The listing builds one solid part. Answer for the finished solid, in the listing's coordinates (mm). A direction names the side the tool comes from. Round coordinates to 2 decimals unless told otherwise and drop trailing zeros. Loops run counter-clockwise (first coordinate to the right, second up) from the corner with the lowest first, then second, coordinate; pieces in that order, holes last. Notation, with made-up numbers: M -9.75,49 L 48.25,49 A13 ccw 48.25,57 Z; hole C 55,71 d4. An arc over 180 degrees is marked long. Answer as a JSON object with one key per item and string values.
```python
from build123d import *

# Parameters (mm, degrees)
F1_DEPTH       = 10
F3_D           = 3.7973
F3_CSINK_D     = 7.7978
F3_CSINK_ANGLE = 82
F4_SIZE        = 5
F5_R           = 5
F6_R           = 15


with BuildPart() as f1:
    # F0 (on Front) → F1 (new body, symmetric)
    with BuildSketch(Plane.XZ):
        with BuildLine():
            Line((0, -15), (0, 15))
            ThreePointArc((0, 15), (-2.4851818051, 16.4611506644), (-5, 17.8706822588))
            Line((-5, 17.8706822588), (-5, 14.2103387279))
            Line((-5, 14.2103387279), (-5, -14.2103387279))
            Line((-5, -14.2103387279), (-5, -17.8706822588))
            ThreePointArc((-5, -17.8706822588), (-2.4851818051, -16.4611506644), (0, -15))
        make_face()
        with BuildLine():
            Line((0, 15), (0, 65))
            Line((0, 65), (-5, 65))
            Line((-5, 65), (-5, 17.8706822588))
            ThreePointArc((-5, 17.8706822588), (-2.4851818051, 16.4611506644), (0, 15))
        make_face()
        with BuildLine():
            Line((0, -65), (0, -15))
            ThreePointArc((0, -15), (-2.4851818051, -16.4611506644), (-5, -17.8706822588))
            Line((-5, -17.8706822588), (-5, -65))
            Line((-5, -65), (0, -65))
        make_face()
        with BuildLine():
            Line((-5, 14.2103387279), (-5, 17.8706822588))
            ThreePointArc((-5, 17.8706822588), (-72.3928986571, 34.9994712149), (-139.6904967398, 17.5))
            ThreePointArc((-139.6904967398, 17.5), (-147.231014529, 10.1554893712), (-150, 0))
            ThreePointArc((-150, 0), (-147.231014529, -10.1554893712), (-139.6904967398, -17.5))
            ThreePointArc((-139.6904967398, -17.5), (-72.3928986571, -34.9994712149), (-5, -17.8706822588))
            Line((-5, -17.8706822588), (-5, -14.2103387279))
            ThreePointArc((-5, -14.2103387279), (-71.5057739854, -31.7990733195), (-138.1393945883, -14.7010569646))
            ThreePointArc((-138.1393945883, -14.7010569646), (-144.4738849633, -8.5312244428), (-146.8, 0))
            ThreePointArc((-146.8, 0), (-144.4738849633, 8.5312244428), (-138.1393945883, 14.7010569646))
            ThreePointArc((-138.1393945883, 14.7010569646), (-71.5057739854, 31.7990733195), (-5, 14.2103387279))
        make_face()
    extrude(amount=F1_DEPTH, both=True)

    # F3 (through all)
    with Locations(Plane(origin=(-5, 0, 0), x_dir=(0, -1, 0), z_dir=(-1, 0, 0))):
        with Locations((0, 55), (0, -55)):
            CounterSinkHole(F3_D / 2, F3_CSINK_D / 2, counter_sink_angle=F3_CSINK_ANGLE)

    # F4
    f4_edges = [f1.edges().sort_by_distance(p)[0] for p in [
        (-2.5, -10, 65),
        (-2.5, 10, 65),
        (-2.5, -10, -65),
        (-2.5, 10, -65),
    ]]
    chamfer(f4_edges, length=F4_SIZE)

    # F5
    f5_edges = [f1.edges().sort_by_distance(p)[0] for p in [
        (-2.5, -5, -65),
        (-2.5, 5, -65),
        (-2.5, -5, 65),
        (-2.5, 5, 65),
    ]]
    fillet(f5_edges, radius=F5_R)

    # F6
    f6_edges = [f1.edges().sort_by_distance(p)[0] for p in [
        (-5, 0, 14.210339),
        (-5, 0, 17.870682),
        (-5, 0, -17.870682),
        (-5, 0, -14.210339),
    ]]
    fillet(f6_edges, radius=F6_R)


solid = f1.part
```
Item 1: The part is cut by section A-A (z = -55). Give the vertices of the cut face in (x, y), then the cut area to 3 significant figures.
Values follow:
{"outline": "M -5,-10 L 0,-10 L 0,-1.9 L -2.7,-1.9 L -5,-3.9 Z; M -5,3.9 L -2.7,1.9 L 0,1.9 L 0,10 L -5,10 Z", "area": "76.4 mm^2"}
Item 2: Flat-ended cylindrical pins translate along their axes: P1, Ø8, axis at y = 6.5, z = -12, coming from the -X side; P2, Ø8, axis at y = -2.5, z = -51, coming from the -X side; P3, Ø6, axis at y = -6, z = 5, coming from the -X side. Find the tip coordinate at first contact, or state that the pin passes through.
Values follow:
{"P1": "x = -148.33", "P2": "x = -5", "P3": "x = -149.9"}
Item 3: The part is cut by section B-B (x = -19). Give the vertices of the cut face in (y, z).
Values follow:
{"outline": "M -10,-26.02 L 10,-26.02 L 10,-21.08 L -10,-21.08 Z; M -10,21.08 L 10,21.08 L 10,26.02 L -10,26.02 Z"}
Item 4: Determine the mould class of faces 4 (the face through (-84.204, -0.14, -34.466)), 5 (the face through (-7.26, 0.14, 13.02)), 6 (the face through (-11.196, -0.14, 28.847)) for opening direction Z: released by +Z, released by -Z, zero draft, split by the parting line, or undercut.
Values follow:
{"face 4": "released by -Z", "face 5": "undercut", "face 6": "released by +Z"}
Item 5: Which of the six approach directions +Z, -Z, +X, -X, +Y, -Y give full straight-line access (tool end or side, diameter ignored) to faces 1 (the face through (-5, 0, 50)), 2 (the face through (-7.26, -0.14, -13.02)), 3 (the face through (-5, 0, -50))?
Values follow:
{"face 1": "+Z, -X, +Y, -Y", "face 2": "+Y, -Y", "face 3": "-Z, -X, +Y, -Y"}
Item 6: Straight lines are drawn through the part: line 1 (Z direction, x = -0.55, y = 0); line 2 (Y direction, x = -1.4, z = 55); line 3 (Z direction, x = -127.5, y = 8.5). For each, find the intervals that lie inside material, in ascending order.
Values follow:
{"line 1": "-65 to -56.9, -53.1 to 53.1, 56.9 to 65", "line 2": "-10 to -1.9, 1.9 to 10", "line 3": "-23.5 to -20, 20 to 23.5"}
Item 7: The part is cut by section D-D (x = -131.5). Give the vertices of the cut face in (y, z).
Values follow:
{"outline": "M -10,-21.69 L 10,-21.69 L 10,-18.15 L -10,-18.15 Z; M -10,18.15 L 10,18.15 L 10,21.69 L -10,21.69 Z"}
Item 8: The part is cut by section C-C (y = 0). Give the vertices of the cut face in (x, z).
Values follow:
{"outline": "M -139.69,-17.5 A139.63 ccw -25.05,-26.87 A15 cw -5,-40.99 L -5,-51.1 L -2.7,-53.1 L 0,-53.1 L 0,53.1 L -2.7,53.1 L -5,51.1 L -5,40.99 A15 cw -25.05,26.87 A139.63 ccw -139.69,17.5 A20.01 ccw Z; M -5,-65 L 0,-65 L 0,-56.9 L -2.7,-56.9 L -5,-58.9 Z; M -5,58.9 L -2.7,56.9 L 0,56.9 L 0,65 L -5,65 Z; hole M -138.14,-14.7 A136.43 ccw -13.58,-18.65 A15 ccw -5,-5.1 L -5,5.1 A15 ccw -13.58,18.65 A136.43 ccw -138.14,14.7 A16.81 ccw Z"}
